The figure shows three views and two pictorial views of one solid part (mm, origin at its lowest corner). Answer the questions. A direction names the side the tool comes from. Give positions to 0.01 mm unless a question says otherwise; leave off trailing zeros. Loops run counter-clockwise (first coordinate to the right, second up) from the corner with the lowest first, then second, coordinate; pieces in that order, holes last. Notation, with made-up numbers: M 2.5,11 L 6.5,11 A20 cw 6.5,36 Z; hole C -35.5,53.5 d9. An arc over 180 degrees is marked long. Write item = value, one per line. Start each with the question number.
1. Section C-C on z = 13.25 is taken. Determine the outline of the cut face in (x, y), plus the area to 3 significant figures.
2. Section B-B on y = 16.5 is taken. Determine the outline of the cut face in (x, z).
3. Flat-ended cylindrical pins translate along their axes: pin 1 Ø8 at (x, z) = (2.5, 11) entering from +Y; pin 2 Ø1 at (x, y) = (8.5, 32.5) entering from +Z; pin 3 Ø1.4 at (y, z) = (12, 21.5) entering from +X. Find the tip coordinate at first contact, or state that the pin passes through.
4. Section A-A on x = 11 is taken. Determine the outline of the cut face in (y, z), plus the area to 3 significant figures.
5. The mould has two halves that part along X. Classify the marked faces 1, 2, 3 and 4: released by +X, released by -X, zero draft, split by the parting line, or undercut.
6. For the marked faces 5, 6 and 7, determine the directions among +Z, -Z, +X, -X, +Y, -Y from which every point of the face is accessible in a straight line to the end or side of a thin tool.
7. Consider L1, parallel to Y at x = 8, z = 21.5; L2, parallel to Z at x = 11.25, y = 4.5; L3, parallel to X at y = 16.5, z = 21. Determine where each line is inside the solid, lowest interval first. Write a range as [from, to].
8. Section D-D on x = 15 is taken. Determine the outline of the cut face in (y, z), plus the area to 3 significant figures.
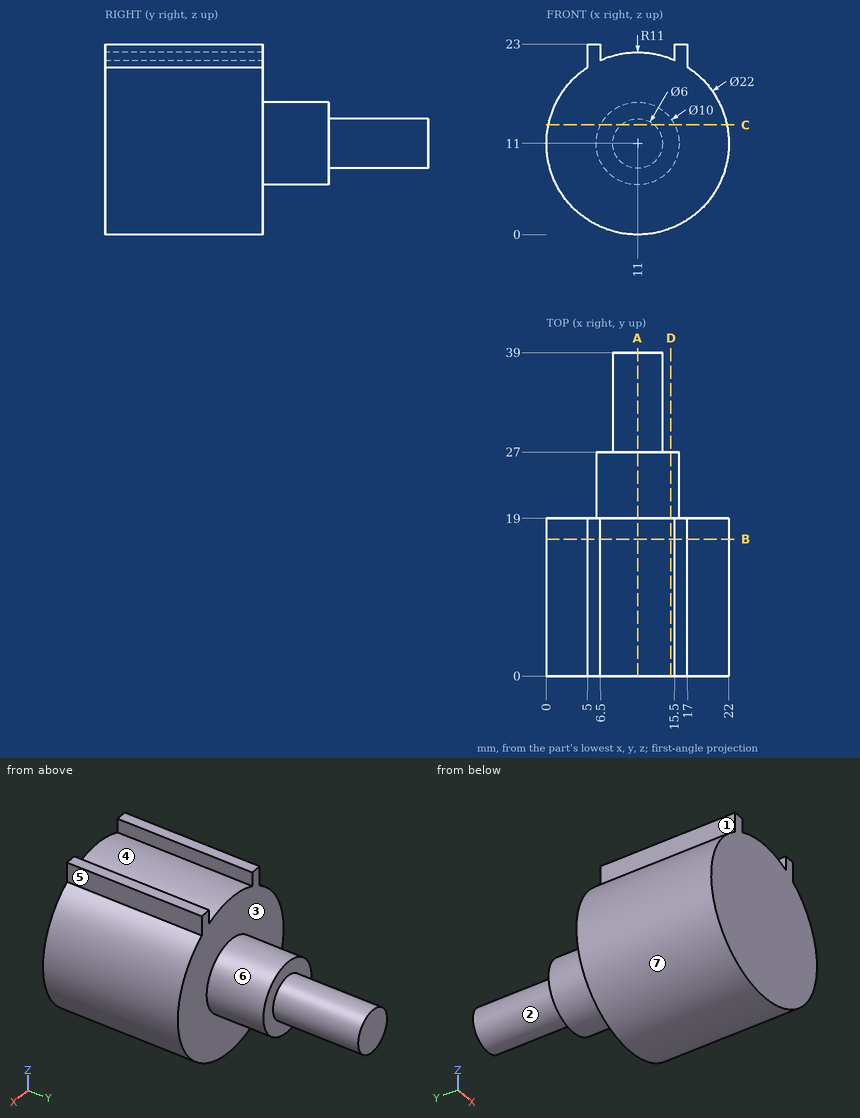
Verdict:
q1.outline = M 0.23,0 L 21.77,0 L 21.77,19 L 15.47,19 L 15.47,27 L 12.98,27 L 12.98,39 L 9.02,39 L 9.02,27 L 6.53,27 L 6.53,19 L 0.23,19 Z
q1.area = 528 mm2
q2.outline = M 5,20.22 A11 ccw long 17,20.22 L 17,23 L 15.5,23 L 15.5,21.04 A11 ccw 6.5,21.04 L 6.5,23 L 5,23 Z
q3.pin_1 = 27
q3.pin_2 = 13.24
q3.pin_3 = 17
q4.outline = M 0,0 L 19,0 L 19,6 L 27,6 L 27,8 L 39,8 L 39,14 L 27,14 L 27,16 L 19,16 L 19,22 L 0,22 Z
q4.area = 570 mm2
q5.face_1 = released by -X
q5.face_2 = split by the parting line
q5.face_3 = zero draft
q5.face_4 = undercut
q6.face_5 = +Z, +X, +Y, -Y
q6.face_6 = +Y
q6.face_7 = +Y, -Y
q7.L1 = [0, 19]
q7.L2 = [0, 22]
q7.L3 = [5, 17]
q8.outline = M 0,0.75 L 19,0.75 L 19,8 L 27,8 L 27,14 L 19,14 L 19,21.25 L 0,21.25 Z
q8.area = 437 mm2
